from build123d import *

# Parameters (mm, degrees)
SKETCH1_W                = 17.8
SKETCH1_H                = 6.2
BOSS_EXTRUDE1_DEPTH      = 5.4
SHELL1_T                 = -1.2
SKETCH2_W                = 6
SKETCH2_H                = 4.2
REVOLVE1_DEPTH           = 8
SKETCH5_W                = 1.864108749
SKETCH5_H                = 2.6
CUT_EXTRUDE1_DEPTH       = 5.4
SKETCH6_W                = 5.2
SKETCH6_H                = 1.6
CUT_EXTRUDE2_DEPTH       = 2.7
SKETCH7_R                = 1.5
BOSS_EXTRUDE2_DEPTH      = 3.8
SKETCH8_W                = 1.2
SKETCH8_H                = 3
BOSS_EXTRUDE3_DEPTH      = 1.4
CHAMFER1_SIZE            = 0.5
CHAMFER1_OF_MIRROR1_SIZE = 0.5
SKETCH9_W                = 5.3
SKETCH9_H                = 2.5
CUT_EXTRUDE3_DEPTH       = 5


# Read off the part's stored shape, not the designer's step: Revolve1
with BuildPart() as part:
    # Sketch1 → Boss-Extrude1 (new body)
    with BuildSketch(Plane(origin=(0, 0, 0), x_dir=(1, 0, 0), z_dir=(0, 1, 0))):
        Rectangle(SKETCH1_W, SKETCH1_H)
    extrude(amount=BOSS_EXTRUDE1_DEPTH)

    # Shell1
    shell1_openings = [part.faces().sort_by_distance(p)[0] for p in [
        (0, 2.7, 3.1),
    ]]
    offset(amount=SHELL1_T, openings=shell1_openings, kind=Kind.INTERSECTION)

    # Sketch2 → Cut-Revolve1 (revolve, cut)
    with BuildSketch(Plane.XY.offset(3.1)):
        with Locations((3, 3.3)):
            Rectangle(SKETCH2_W, SKETCH2_H)
    revolve(axis=Axis((0, 1.2, 3.1), (0, 1, 0)), mode=Mode.SUBTRACT)

    # Revolve1 outline → Revolve1 (add)
    with BuildSketch(Plane(origin=(0, 0, 0), x_dir=(1, 0, 0), z_dir=(0, 1, 0))):
        with BuildLine():
            Line((-5.180733539, 1.9), (-3.31662479, 1.9))
            ThreePointArc((-3.31662479, 1.9), (0, 2.9), (3.31662479, 1.9))
            Line((3.31662479, 1.9), (5.180733539, 1.9))
            ThreePointArc((5.180733539, 1.9), (0, 4.1), (-5.180733539, 1.9))
        make_face()
    extrude(amount=REVOLVE1_DEPTH)

    # Sketch5 → Cut-Extrude1 (cut)
    with BuildSketch(Plane.XY.offset(-1.9)):
        with Locations((-4.248679165, 6.7)):
            Rectangle(SKETCH5_W, SKETCH5_H)
        with Locations((4.248679165, 6.7)):
            Rectangle(SKETCH5_W, SKETCH5_H)
    extrude(amount=-CUT_EXTRUDE1_DEPTH, mode=Mode.SUBTRACT)

    # Sketch6 → Cut-Extrude2 (cut, symmetric)
    with BuildSketch(Plane(origin=(0, 0, -3.1), x_dir=(-1, 0, 0), z_dir=(0, 0, -1))):
        with Locations((0, 2)):
            Rectangle(SKETCH6_W, SKETCH6_H)
    extrude(amount=CUT_EXTRUDE2_DEPTH, both=True, mode=Mode.SUBTRACT)

    # Sketch7 → Boss-Extrude2 (add)
    with BuildSketch(Plane(origin=(0, 0, -3.1), x_dir=(-1, 0, 0), z_dir=(0, 0, -1))):
        with Locations(Location((6.1, 3.4, 0), (0, 0, 180))):
            Circle(SKETCH7_R)
        with Locations(Location((-6.1, 3.4, 0), (0, 0, 180))):
            Circle(SKETCH7_R)
    extrude(amount=BOSS_EXTRUDE2_DEPTH)

    # Sketch8 → Boss-Extrude3 (add)
    with BuildSketch(Plane.ZY.offset(-7.7)):
        with Locations((3.7, 2.7)):
            Rectangle(SKETCH8_W, SKETCH8_H)
    boss_extrude3 = extrude(amount=-BOSS_EXTRUDE3_DEPTH)

    # Chamfer1
    chamfer1_edges = [part.edges().sort_by_distance(p)[0] for p in [
        (9.1, 2.7, 4.3),
    ]]
    chamfer(chamfer1_edges, length=CHAMFER1_SIZE)

    # Mirror1: Boss-Extrude3 across plane
    add(boss_extrude3.mirror(Plane(origin=(0, 0, 0), x_dir=(0, 0, 1), z_dir=(1, 0, 0))))

    # Chamfer1 of Mirror1
    chamfer1_of_mirror1_edges = [part.edges().sort_by_distance(p)[0] for p in [
        (-9.1, 2.7, 4.3),
    ]]
    chamfer(chamfer1_of_mirror1_edges, length=CHAMFER1_OF_MIRROR1_SIZE)

    # Sketch9 → Cut-Extrude3 (cut, symmetric)
    with BuildSketch(Plane(origin=(0, 1.2, 0), x_dir=(1, 0, 0), z_dir=(0, 1, 0))):
        with Locations((0, -1.85)):
            Rectangle(SKETCH9_W, SKETCH9_H)
    extrude(amount=CUT_EXTRUDE3_DEPTH, both=True, mode=Mode.SUBTRACT)


solid = part.part
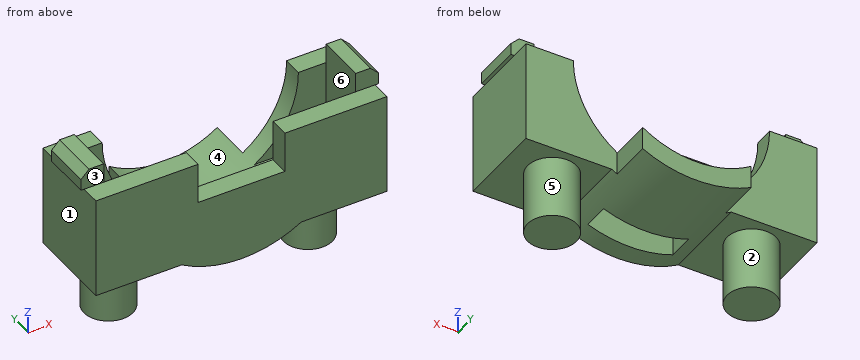
Verification items for the finished model (mm, model axes). Face numbers are marked on the shaded views. A direction names the side the tool comes from. Coordinates: 2 decimals unless noted, no trailing zeros. Loops run counter-clockwise (first coordinate to the right, second up) from the corner with the lowest first, then second, coordinate; pieces in that order, holes last. Notation, with made-up numbers: (74.5, -32) -> (87.5, -32) arc R16 cw to (87.5, -11) -> close; hole circle Ø3 at (-27.5, 14). An arc over 180 degrees is marked (long way). Answer as CSV lines item,"result".
1) Cross-section at A-A, the plane x = 0.25. Record the cut outline in (y, z), then the cut area to 3 significant figures.
Found:
outline,"(0, -4.1) -> (1.2, -4.1) -> (1.2, 0.6) -> (0, 0.6) -> close; (2.8, -4.1) -> (8, -4.1) -> (8, -2.89) -> (2.8, -2.89) -> close"
area,"11.9 mm2"
2) Release check for a two-part mould opening along X. For the marked faces 1, 2 and 3 record: +X half, -X half, draft (parallel to the pull), parting line (faces both ways), or undercut.
Found:
face 1,"-X half"
face 2,"undercut"
face 3,"draft"
3) Thickness scan on L1, parallel to X at y = 3.5, z = 3.5; L2, parallel to Y at x = 1.25, z = -3; L3, parallel to X at y = 3.75, z = 1. Record the ranges inside material, lowest first. Write a range as from..to.
Found:
L1,"x = -9.1..-7.7, 7.7..9.1"
L2,"y = 0..1.2, 2.8..8"
L3,"x = -8.9..-7.7, 7.7..8.9"
4) Depth check by flat-ended pin: pin 1 (0.6 mm diameter, centred on x = -8.5, z = 4, fed in from +Y); pin 2 (0.9 mm diameter, centred on y = 3, z = 1.5, fed in from -X); pin 3 (1 mm diameter, centred on x = 4.5, z = -4.5, fed in from -Y). Enter the tip coordinate at first touch or a pass-through.
Found:
pin 1,"stops at y = 4.2"
pin 2,"stops at x = -8.9"
pin 3,"stops at y = 2.38"
5) Cross-section at D-D, the plane z = -1. Record the cut outline in (x, y), then the cut area to 3 significant figures.
Found:
outline,"(-8.9, 0) -> (8.9, 0) -> (8.9, 5.4) -> (4.38, 5.4) -> (4.38, 4.2) -> (7.7, 4.2) -> (7.7, 1.2) -> (-7.7, 1.2) -> (-7.7, 4.2) -> (-4.38, 4.2) -> (-4.38, 5.4) -> (-8.9, 5.4) -> close"
area,"39.4 mm2"
6) Tool access check on the marked faces 4, 5 and 6. Record the directions out of +Z, -Z, +X, -X, +Y, -Y that give a thin tool (end or side, any length) a straight path to the whole face; none if there is none.
Found:
face 4,"+Z, +Y"
face 5,"-Z"
face 6,"+Z"
7) Cross-section at B-B, the plane z = -6. Record the cut outline in (x, y), then the cut area to 3 significant figures.
Found:
outline,"circle Ø3 at (-6.1, 3.4); circle Ø3 at (6.1, 3.4)"
area,"14.1 mm2"
8) Cross-section at C-C, the plane y = 3.4. Record the cut outline in (x, z), then the cut area to 3 significant figures.
Found:
outline,"(-9.1, 3.1) -> (-8.9, 3.1) -> (-8.9, -3.1) -> (-7.6, -3.1) -> (-7.6, -6.9) -> (-4.6, -6.9) -> (-4.6, -3.1) -> (-3.66, -3.1) arc R7.2 ccw to (3.66, -3.1) -> (4.6, -3.1) -> (4.6, -6.9) -> (7.6, -6.9) -> (7.6, -3.1) -> (8.9, -3.1) -> (8.9, 3.1) -> (9.1, 3.1) -> (9.1, 3.8) -> (8.6, 4.3) -> (7.7, 4.3) -> (7.7, -1.9) -> (3.32, -1.9) arc R6 cw to (-3.32, -1.9) -> (-7.7, -1.9) -> (-7.7, 4.3) -> (-8.6, 4.3) -> (-9.1, 3.8) -> close"
area,"59.7 mm2"
